Input: part model. Units: mm. Frame: model coordinates. Face numbers are marked on the shaded views. Coordinates: 2 decimals unless noted, no trailing zeros. Order: outer loops, then holes, each group sorted by start corner. A loop starts at its lowest first (then second) coordinate and runs counter-clockwise, first axis right, second up. Notation, with made-up numbers: M 24.5,-10 L 81.5,-10 A16 ccw 81.5,10 Z; hole C 62,56.5 d6. An arc over 180 degrees is marked long. One line per item, written item: value.
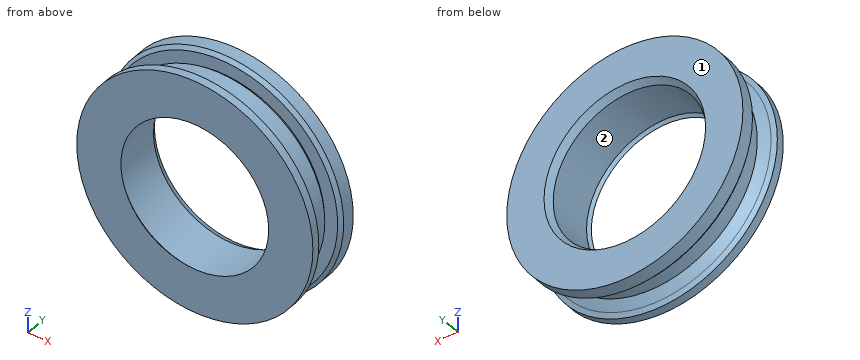
Autodesk Inventor part; units mm, degrees
ref_plane "YZ Plane" through (0, 0, 0) normal (1, 0, 0) x (0, 1, 0)
ref_plane "XZ Plane" through (0, 0, 0) normal (0, 1, 0) x (-1, 0, 0)
ref_plane "XY Plane" through (0, 0, 0) normal (0, 0, 1) x (1, 0, 0)
sketch "Sketch1" plane through (0, 0, 0) normal (0, 0, 1) x (1, 0, 0)
  line L0 (11.1, 0) -> (17.1, 0)
  line L1 (17.1, 0) -> (17.1, 8) construction
  line L2 (17.1, 8) -> (11.1, 8) construction
  line L3 (11.1, 8) -> (11.1, 0) construction
  line L4 (0, 0) -> (0, 7.3935) construction
  line L5 (17.1, 8) -> (17.1, 6.8284)
  line L6 (17.1, 1.1716) -> (17.1, 0)
  circle A0 centre (18.1, 4) radius 3
  line L7 (15.1, 5.6) -> (15.1, 2.4) construction
  line L8 (15.1, 2.4) -> (16.4287, 1.5087)
  line L9 (14.7, 5.6) -> (16.6, 5.6)
  line L10 (16.6, 5.6) -> (17.1, 6.1)
  line L11 (17.1, 6.1) -> (17.1, 6.8284)
  line L12 (14.7, 5.6) -> (15.1, 5.1)
  line L13 (15.1, 5.1) -> (15.1, 2.4)
  line L14 (11.7, 8) -> (11.1, 7)
  line L15 (11.1, 0.4) -> (10.7, 0)
  line L16 (10.7, 0) -> (11.1, 0)
  line L17 (11.7, 8) -> (17.1, 8)
  line L18 (11.1, 7) -> (11.1, 0.4)
  point P0 (17.1, 4)
  point P1 (15.5286, 5.5452)
  point P2 (15.5286, 2.4548)
  point P3 (15.1, 4)
  point P4 (16.3509, 6.4373)
  dimension "d13" = 6
  dimension "d6" = 8
  dimension "d7" = 11.1
  dimension "d12" = 1
  dimension "d14" = 6
  dimension "d17" = 3.2
  dimension "d18" = 1.9
  dimension "d19" = 135
  dimension "d24" = 0.5
  dimension "d25" = 0.5
  dimension "d27" = 0.6
  dimension "d28" = 1
  dimension "d29" = 0.4
  dimension "d30" = 0.4
revolve "Revolution1" add sketch "Sketch1" angle 360 about axis through (0, 0, 0) along (0, 1, 0) picked at (16.0469, 5.7737) contours L16 L15 L18 L14 L17 L5 A0 L9 L12 L13 L8 L6 L0 | L11 L10 L9 A0
properties part number "pully 16mmx30mmx6mm"
(1) First-contact query: pin 1 (2 mm diameter, centred on y = 2, z = -5, fed in from -X); pin 2 (4 mm diameter, centred on x = -10.5, z = 11.5, fed in from -Y); pin 3 (1.5 mm diameter, centred on x = 1.5, y = 6, fed in from -Z); pin 4 (2 mm diameter, centred on x = -7.5, y = 6.5, fed in from -Z). Flat tips, straight axial feed; report the tip coordinate or a pass-through.
Data:
pin 1: stops at x = -16.51
pin 2: stops at y = 0
pin 3: stops at z = -17.08
pin 4: stops at z = -15.82
(2) Cut plane A-A on x = 0. Output: boundary loops of the cut face in (y, z).
Data:
outline: M 0,-17.1 L 1.17,-17.1 A3 cw 1.51,-16.43 L 2.4,-15.1 L 5.1,-15.1 L 5.6,-14.7 L 5.6,-16.6 L 6.1,-17.1 L 8,-17.1 L 8,-11.7 L 7,-11.1 L 0.4,-11.1 L 0,-10.7 Z; M 0,10.7 L 0.4,11.1 L 7,11.1 L 8,11.7 L 8,17.1 L 6.1,17.1 L 5.6,16.6 L 5.6,14.7 L 5.1,15.1 L 2.4,15.1 L 1.51,16.43 A3 cw 1.17,17.1 L 0,17.1 Z
(3) Ray query, line 1 (Z direction, x = 0, y = 2.5); line 2 (Z direction, x = 8, y = 3.75). Return the intervals inside material, ascending. Write a range as from..to.
Data:
line 1: z = -15.1..-11.1, 11.1..15.1
line 2: z = -12.81..-7.69, 7.69..12.81
(4) Draft query along Z for the marked faces 1 and 2. Return one class per face: released by +Z, released by -Z, zero draft, split by the parting line, or undercut.
Data:
face 1: zero draft
face 2: undercut
(5) Cut plane B-B on z = 0. Output: boundary loops of the cut face in (x, y), plus the area to 3 significant figures.
Data:
outline: M -17.1,0 L -10.7,0 L -11.1,0.4 L -11.1,7 L -11.7,8 L -17.1,8 L -17.1,6.1 L -16.6,5.6 L -14.7,5.6 L -15.1,5.1 L -15.1,2.4 L -16.43,1.51 A3 cw -17.1,1.17 Z; M 10.7,0 L 17.1,0 L 17.1,1.17 A3 cw 16.43,1.51 L 15.1,2.4 L 15.1,5.1 L 14.7,5.6 L 16.6,5.6 L 17.1,6.1 L 17.1,8 L 11.7,8 L 11.1,7 L 11.1,0.4 Z
area: 79.7 mm2
